For this review, take the finished solid that the model builds, in its own axes (mm). A direction names the side the tool comes from. Coordinates: 2 decimals unless noted, no trailing zeros. Loops run counter-clockwise (first coordinate to the right, second up) from the corner with the lowest first, then second, coordinate; pieces in that order, holes last.
1. Take a section at A-A, the plane y = -1715. State the section outline as (x, z) points, then the cut area to 3 significant figures.
2. Take a section at B-B, the plane x = 6277. State the section outline as (y, z) points, then the cut area to 3 significant figures.
3. Take a section at C-C, the plane z = -571. State the section outline as (x, y) points.
4. Take a section at D-D, the plane x = 6419. State the section outline as (y, z) points.
5. Machinability: for faces 1 (the face through (6223, -1634, 13)), 2 (the face through (6329, -1524, -801)), 3 (the face through (6329, -1524, 798)), which of the approach directions +Z, -Z, +X, -X, +Y, -Y give a long, thin tool a straight path to every point of the face, cutting with its end or side? Answer none if there is none.
6. Clearance check with flat-ended pins moving along their axes: P1, Ø1.5, axis at x = 6326, y = -1711, coming from the +Z side; P2, Ø12, axis at x = 6334.5, y = -1592, coming from the +Z side; P3, Ø12, axis at x = 6274.5, y = -1522.5, coming from the +Z side. State where each tip first meets the part, or that it passes through.
7. To check wall thickness, follow probe 1 along Y at (x, z) = (6282.5, -729.5); probe 2 along Z at (x, y) = (6299, -1585.5); probe 3 along Z at (x, y) = (6418.5, -1661.5). State the ranges of each line that lie inside material, in increasing order.
```python
from build123d import *

# Parameters (mm, degrees)
F0_W     = 304.8
F0_H     = 355.6
F1_DEPTH = 952.5
F3_DEPTH = 355.601
F4_W     = 575.44121
F4_H     = 4171.496656
F5_DEPTH = 241.301
F7_DEPTH = 241.301
F9_DEPTH = 241.301


with BuildPart() as f1:
    # F0 (on Top) → F1 (new body, symmetric)
    with BuildSketch(Plane.XY):
        with Locations((6375.4, -1600.2)):
            Rectangle(F0_W, F0_H)
    extrude(amount=F1_DEPTH, both=True)

    # F2 (on face) → F3 (cut, through all)
    with BuildSketch(Plane.XZ.offset(1778)):
        Polygon((6369.221802, 914.017151), (6435.014533, 762), (6464.3, 203.2), (6464.3, 0), (6464.3, -203.2), (6435.014533, -762), (6369.221802, -914.017151), (6223, -939.8), (6223, -1333.5), (8458.2, -1333.5), (8458.2, 1333.5), (6223, 1333.5), (6223, 939.8), align=None)
    extrude(amount=-F3_DEPTH, mode=Mode.SUBTRACT)

    # F4 (on face) → F5 (cut, through all)
    with BuildSketch(Plane(origin=(6223, 0, 0), x_dir=(0, -1, 0), z_dir=(-1, 0, 0))):
        with Locations((2028.890605, 152.959056)):
            Rectangle(F4_W, F4_H)
    extrude(amount=-F5_DEPTH, mode=Mode.SUBTRACT)

    # F6 (on face) → F7 (cut, through all)
    with BuildSketch(Plane(origin=(6223, 0, 0), x_dir=(0, -1, 0), z_dir=(-1, 0, 0))):
        Polygon((1422.4, -939.8), (1422.4, 0), (1422.4, 939.8), (1524, 939.8), (1524, 1382.621926), (624.785322, 1382.621926), (624.785322, -1382.621926), (1524, -1382.621926), (1524, -939.8), align=None)
        Polygon((1460.5, -152.4), (1460.5, 0), (1422.4, 0), (1422.4, -939.8), (1524, -939.8), (1524, -711.2), align=None)
        Polygon((1422.4, 0), (1460.5, 0), (1460.5, 152.4), (1524, 711.2), (1524, 939.8), (1422.4, 939.8), align=None)
    extrude(amount=-F7_DEPTH, mode=Mode.SUBTRACT)

    # F8 (on face) → F9 (cut, through all)
    with BuildSketch(Plane(origin=(6223, 0, 0), x_dir=(0, -1, 0), z_dir=(-1, 0, 0))):
        Polygon((1753.895535, 1074.559246), (1407.100362, 1074.559246), (1407.100362, 825.20454), (1582.42, 918.423645), (1664.97, 927.1), (1753.895535, 927.1), align=None)
        Polygon((1753.895535, -1074.559246), (1753.895535, -927.1), (1664.97, -927.1), (1582.42, -918.423645), (1407.100362, -825.20454), (1407.100362, -1074.559246), align=None)
    extrude(amount=-F9_DEPTH, mode=Mode.SUBTRACT)


solid = f1.part
```
Results list:
1. outline: (6223, -927.1) - (6295.03, -927.1) - (6369.22, -914.02) - (6435.01, -762) - (6464.3, -203.2) - (6464.3, 203.2) - (6435.01, 762) - (6369.22, 914.02) - (6295.03, 927.1) - (6223, 927.1) - close
1. area: 409,000 mm2
2. outline: (-1741.17, -927.1) - (-1664.97, -927.1) - (-1582.42, -918.42) - (-1524, -887.36) - (-1524, -711.2) - (-1460.5, -152.4) - (-1460.5, 152.4) - (-1524, 711.2) - (-1524, 887.36) - (-1582.42, 918.42) - (-1664.97, 927.1) - (-1741.17, 927.1) - close
2. area: 454,000 mm2
3. outline: (6223, -1741.17) - (6445.02, -1741.17) - (6445.02, -1508.07) - (6223, -1508.07) - close
4. outline: (-1741.17, -799) - (-1524, -799) - (-1524, -711.2) - (-1460.5, -152.4) - (-1460.5, 152.4) - (-1524, 711.2) - (-1524, 799) - (-1741.17, 799) - close
5. face 1: +Z, -Z, -X, +Y, -Y
5. face 2: -Z, +X, -X, +Y
5. face 3: +Z, +X, -X, +Y
6. P1: stops at z = 921.77
6. P2: stops at z = 920.06
6. P3: stops at z = 889.75
7. probe 1: y = -1741.17 to -1524
7. probe 2: z = -918.75 to 918.75
7. probe 3: z = -800.16 to 800.16
